Build history of the part. All positions in model axes, mm. Face numbers are marked on the shaded views. Coordinates: 2 decimals unless noted, no trailing zeros. Order: outer loops, then holes, each group sorted by start corner. A loop starts at its lowest first (then second) coordinate and runs counter-clockwise, first axis right, second up. Notation, with made-up numbers: M -9,-4.75 L -1,-4.75 A11 ccw -1,16.25 Z; hole C -1.75,19.5 d5. An arc over 180 degrees is marked long. Write item = value, one per line. Start each with the question number.
Q1. Drill centre lines: probe 1 along X at (y, z) = (-6.5, 0.5); probe 2 along X at (y, z) = (-2.75, -2.75); probe 3 along Y at (x, z) = (-19, -10). Where is each one in solid material? Low to high.
Q2. Pull direction X, two halves, no side cores. Call the marked faces 1, 2 and 3: released by +X, released by -X, zero draft, split by the parting line, or undercut.
Q3. Band-saw the part on C-C on y = 15.25. Write the cut outline in (x, z), plus the area to 3 significant figures.
Q4. Band-saw the part on D-D on y = -4. Write the cut outline in (x, z).
Q5. Band-saw the part on A-A on z = 0. Write the cut outline in (x, y).
Q6. Band-saw the part on B-B on x = 0. Write the cut outline in (y, z), plus the area to 3 significant figures.
Q7. Pin check, flat tips, straight feed: P1, Ø7.5, axis at x = 1.5, z = 3, coming from the -Y side; P2, Ø1.5, axis at x = 37.5, z = -7.5, coming from the +Y side; P3, Ø9.5, axis at x = 0, z = 0, coming from the -Y side; P4, Ø16.5, axis at x = -1.5, z = -0.5, coming from the +Y side. Stop position of each tip, or through.
```python
from build123d import *

# Parameters (mm, degrees)
SKETCH1_W           = 100
SKETCH1_H           = 30
BOSS_EXTRUDE1_DEPTH = 20
CUT_EXTRUDE1_DEPTH  = 62.64414003
FILLET1_R           = 5
SKETCH3_W           = 100
SKETCH3_H           = 30
BOSS_EXTRUDE2_DEPTH = 10
SKETCH4_R           = 6
CUT_EXTRUDE2_DEPTH  = 5
SKETCH5_R           = 7.5
CUT_EXTRUDE3_DEPTH  = 4.75
CHAMFER1_SIZE       = 1


with BuildPart() as part:
    # Sketch1 → Boss-Extrude1 (new body)
    with BuildSketch(Plane(origin=(0, 0, 0), x_dir=(1, 0, 0), z_dir=(0, 1, 0))):
        Rectangle(SKETCH1_W, SKETCH1_H)
    extrude(amount=BOSS_EXTRUDE1_DEPTH)

    # Sketch2 → Cut-Extrude1 (cut, through all)
    with BuildSketch(Plane.XY.offset(15)):
        with BuildLine():
            Line((-50, 20), (50, 20))
            ThreePointArc((50, 20), (0, 12), (-50, 20))
        make_face()
    extrude(amount=-CUT_EXTRUDE1_DEPTH, mode=Mode.SUBTRACT)

    # Fillet1
    fillet1_edges = [part.edges().sort_by_distance(p)[0] for p in [
        (-50, 20, 0),
        (50, 20, 0),
    ]]
    fillet(fillet1_edges, radius=FILLET1_R)

    # Sketch3 → Boss-Extrude2 (add)
    with BuildSketch(Plane.XZ):
        Rectangle(SKETCH3_W, SKETCH3_H)
    extrude(amount=BOSS_EXTRUDE2_DEPTH)

    # Sketch4 → Cut-Extrude2 (cut)
    with BuildSketch(Plane.XZ.offset(10)):
        with Locations(Location((0, 0, 0), (0, 0, 270))):
            Circle(SKETCH4_R)
    extrude(amount=-CUT_EXTRUDE2_DEPTH, mode=Mode.SUBTRACT)

    # Sketch5 → Cut-Extrude3 (cut)
    with BuildSketch(Plane.XZ.offset(5)):
        with Locations(Location((0, 0, 0), (0, 0, 270))):
            Circle(SKETCH5_R)
    extrude(amount=-CUT_EXTRUDE3_DEPTH, mode=Mode.SUBTRACT)

    # Chamfer1
    chamfer1_edges = [part.edges().sort_by_distance(p)[0] for p in [
        (0, -10, 6),
    ]]
    chamfer(chamfer1_edges, length=CHAMFER1_SIZE)


solid = part.part
```
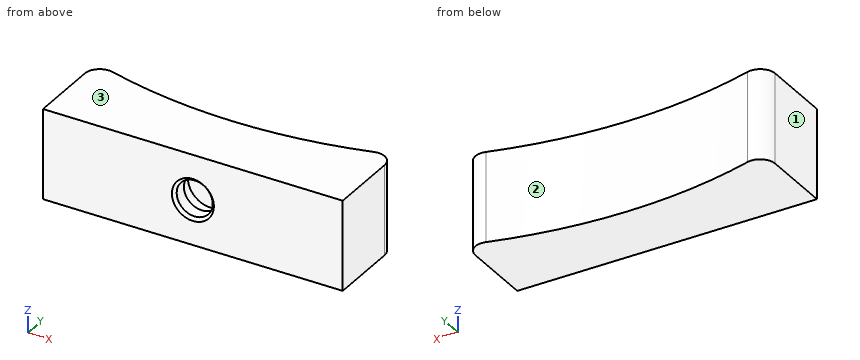
Recorded:
q1.probe_1 = -50 to -5.98, 5.98 to 50
q1.probe_2 = -50 to -6.98, 6.98 to 50
q1.probe_3 = -10 to 13.13
q2.face_1 = released by -X
q2.face_2 = undercut
q2.face_3 = zero draft
q3.outline = M -49.58,-15 L -32.11,-15 L -32.11,15 L -49.58,15 Z; M 32.11,-15 L 49.58,-15 L 49.58,15 L 32.11,15 Z
q3.area = 1,050 mm2
q4.outline = M -50,-15 L 50,-15 L 50,15 L -50,15 Z; hole C 0,0 d15
q5.outline = M -50,-10 L -7,-10 L -6,-9 L -6,-5 L -7.5,-5 L -7.5,-0.25 L 7.5,-0.25 L 7.5,-5 L 6,-5 L 6,-9 L 7,-10 L 50,-10 L 50,13.25 A5 ccw 43.64,18.06 A160.25 cw -43.64,18.06 A5 ccw -50,13.25 Z
q6.outline = M -10,-15 L 12,-15 L 12,15 L -10,15 L -10,7 L -9,6 L -5,6 L -5,7.5 L -0.25,7.5 L -0.25,-7.5 L -5,-7.5 L -5,-6 L -9,-6 L -10,-7 Z
q6.area = 528 mm2
q7.P1 = -10
q7.P2 = 16.63
q7.P3 = -0.25
q7.P4 = 12.3
